```python
from build123d import *

# Parameters (mm, degrees)
F3_R            = 17.272
F4_DEPTH        = 25.4
F5_SIZE         = 6.35
F7_D            = 4.826
F7_COPIES_COUNT = 4


# Not quite as in the source:
# - a pattern or mirror of a feature is missing from the dataset's text; its kind, count and spacing are read off the source's solid


with BuildPart() as f1:
    # F0 (on Front) → F1 (revolve)
    with BuildSketch(Plane.XZ):
        with BuildLine():
            ThreePointArc((0, -25.4), (-17.9605122421, -17.9605122421), (-25.4, 0))
            Line((-25.4, 0), (-38.1, 0))
            Line((-38.1, 0), (-38.1, -31.75))
            Line((-38.1, -31.75), (0, -31.75))
            Line((0, -31.75), (0, -25.4))
        make_face()
    revolve(axis=Axis((0, 0, -28.575), (0, 0, 1)))

    # F3 (on offset) → F4 (cut)
    with BuildSketch(Plane.XY.offset(-37.2872)):
        Circle(F3_R)
    extrude(amount=F4_DEPTH, mode=Mode.SUBTRACT)

    # F5
    f5_edges = [f1.edges().sort_by_distance(p)[0] for p in [
        (-17.272, 0, -31.75),
    ]]
    chamfer(f5_edges, length=F5_SIZE)

    # F7 (through all)
    with Locations(Plane.XY):
        with Locations((0, -34.544)):
            f7 = Hole(F7_D / 2)

    # F7_copies: F7 ×4 about axis
    f7_copies_axis = Axis((0, 0, 0), (0, 0, 1))
    for i in range(1, F7_COPIES_COUNT):
        add(f7.rotate(f7_copies_axis, i * 360 / F7_COPIES_COUNT), mode=Mode.SUBTRACT)


solid = f1.part
```
Verification items for the finished model (mm, model axes). Give positions to 0.01 mm unless a question says otherwise; leave off trailing zeros. Loops run counter-clockwise (first coordinate to the right, second up) from the corner with the lowest first, then second, coordinate; pieces in that order, holes last.
1. Go/stop test with flat-tipped pins: pin 1 Ø12 at (x, z) = (-20.5, -23.5) entering from +Y; pin 2 Ø3 at (x, y) = (34.544, 0) entering from -Z; pin 3 Ø4 at (x, z) = (-21.5, -3.5) entering from +Y; pin 4 Ø2 at (y, z) = (3.5, -5) entering from -X. Record where each tip stops, or that it passes through.
2. Section check A-A, the plane y = 0. Enter the section's corners in (x, z), then the cut area to 3 significant figures.
3. Section check D-D, the plane x = 27. Enter the section's corners in (y, z).
4. Thickness scan on line 1 (Y direction, x = 0, z = -21.5); line 2 (Y direction, x = -0.5, z = -5). Record the ranges inside material, lowest first.
5. Mould release check, pull along Y, two halves, no side actions. Record for faces 1 (the flat face through (-16.4, -17.5, -31.75)), 2 (the cylindrical face through (30.235, 23.183, -16.097)), 3 (the cylindrical face through (-1.3, -32.51, -16.1)), 4 (the cylindrical face through (1.3, 32.51, -16.1)): released by +Y, released by -Y, zero draft, split by the parting line, or undercut.
6. Section check C-C, the plane z = -27. Enter the section's corners in (x, y).
Geometry says:
1. pin 1: stops at y = 35.23
1. pin 2: passes through
1. pin 3: stops at y = 32.73
1. pin 4: stops at x = -38.02
2. outline: (-38.1, -31.75) - (-36.96, -31.75) - (-36.96, 0) - (-38.1, 0) - close; (-32.13, -31.75) - (-23.62, -31.75) - (-17.27, -25.4) - (-17.27, -18.62) arc R25.4 cw to (-25.4, 0) - (-32.13, 0) - close; (17.27, -25.4) - (23.62, -31.75) - (32.13, -31.75) - (32.13, 0) - (25.4, 0) arc R25.4 cw to (17.27, -18.62) - close; (36.96, -31.75) - (38.1, -31.75) - (38.1, 0) - (36.96, 0) - close
2. area: 766 mm2
3. outline: (-26.88, -31.75) - (26.88, -31.75) - (26.88, 0) - (-26.88, 0) - close
4. line 1: y = -38.1 to -36.96, -32.13 to -17.27, 17.27 to 32.13, 36.96 to 38.1
4. line 2: y = -38.1 to -36.9, -32.18 to -24.9, 24.9 to 32.18, 36.9 to 38.1
5. face 1: zero draft
5. face 2: split by the parting line
5. face 3: undercut
5. face 4: undercut
6. outline: circle Ø76.2 at (0, 0); hole circle Ø4.83 at (-34.54, 0); hole circle Ø37.74 at (0, 0); hole circle Ø4.83 at (0, -34.54); hole circle Ø4.83 at (0, 34.54); hole circle Ø4.83 at (34.54, 0)
